Model file for the job. Use its own axes, mm. A direction names the side the tool comes from. Give positions to 0.01 mm unless a question says otherwise; leave off trailing zeros. Order: outer loops, then holes, each group sorted by start corner. A loop starts at its lowest first (then second) coordinate and runs counter-clockwise, first axis right, second up. Notation, with made-up numbers: (22, 68.25) -> (41, 68.25) arc R23 ccw to (41, 102.25) -> close; hole circle Ø4 at (75, -29). An arc over 180 degrees is marked (long way). Answer in a Markdown table with one row per item. Add a question column.
Autodesk Inventor part; units mm, degrees
ref_plane "YZ Plane" through (0, 0, 0) normal (1, 0, 0) x (0, 1, 0)
ref_plane "XZ Plane" through (0, 0, 0) normal (0, 1, 0) x (-1, 0, 0)
ref_plane "XY Plane" through (0, 0, 0) normal (0, 0, 1) x (1, 0, 0)
sketch "Sketch1" plane through (0, 0, 0) normal (0, 0, 1) x (1, 0, 0)
  line L0 (-4, -6.5) -> (4, -6.5)
  line L1 (4, -6.5) -> (4, 6.5)
  line L2 (4, 6.5) -> (-4, 6.5)
  line L3 (-4, 6.5) -> (-4, -6.5)
  line L4 (-4, -6.5) -> (4, 6.5) construction
  line L5 (4, -6.5) -> (-4, 6.5) construction
  point P0 (0, 0)
  dimension "d0" = 13
  dimension "d1" = 8
extrude "Extrusion1" add sketch "Sketch1" against normal blind 9.8
sketch "Sketch2" plane through (0, 0, 0) normal (0, 0, 1) x (1, 0, 0)
  circle A0 centre (0, 0) radius 2.885
  dimension "d4" = 5.77
extrude "Extrusion2" add sketch "Sketch2" along normal blind 8.5
properties part number "switch"
Item 1: Saw through at A-A on x = 0. List the corners of the cut face in (y, z) (3 decimals), plus the area to 3 significant figures.
Item 2: Pin check, flat tips, straight feed: pin 1 Ø6 at (y, z) = (1, 4) entering from +X (3 decimals); pin 2 Ø5 at (y, z) = (3, 6.5) entering from +X. Stop position of each tip, or through.
Item 3: Which spindle directions (+Z, -Z, +X, -X, +Y, -Y) get a long thin tool onto all of the face, cutting with end or side? Do faces 1 (the flat face through (-1, 3, 0)), 2 (the flat face through (0, 0, 8.5)). Say none if no direction does.
Item 4: Saw through at D-D on y = -5.25. List the corners of the cut face in (x, z).
Item 5: Saw through at B-B on y = 0. List the corners of the cut face in (x, z) (3 decimals).
Item 6: Wall check: line 1 (Z direction, x = 1.5, y = 5.75); line 2 (Y direction, x = 0, z = 1.25) (3 decimals); line 3 (X direction, y = 2.5, z = 0.75). Give the ranges that are in metal, low to high.
Item 7: Saw through at C-C on z = 3.5. List the corners of the cut face in (x, y) (3 decimals), plus the area to 3 significant figures.
Evaluation:
| question | item | result |
|---|---|---|
| 1 | outline | (-6.5, -9.8) -> (6.5, -9.8) -> (6.5, 0) -> (2.885, 0) -> (2.885, 8.5) -> (-2.885, 8.5) -> (-2.885, 0) -> (-6.5, 0) -> close |
| 1 | area | 176 mm2 |
| 2 | pin 1 | stops at x = 2.885 |
| 2 | pin 2 | stops at x = 2.84 |
| 3 | face 1 | +Z |
| 3 | face 2 | +Z, +X, -X, +Y, -Y |
| 4 | outline | (-4, -9.8) -> (4, -9.8) -> (4, 0) -> (-4, 0) -> close |
| 5 | outline | (-4, -9.8) -> (4, -9.8) -> (4, 0) -> (2.885, 0) -> (2.885, 8.5) -> (-2.885, 8.5) -> (-2.885, 0) -> (-4, 0) -> close |
| 6 | line 1 | z = -9.8 to 0 |
| 6 | line 2 | y = -2.885 to 2.885 |
| 6 | line 3 | x = -1.44 to 1.44 |
| 7 | outline | circle Ø5.77 at (0, 0) |
| 7 | area | 26.1 mm2 |
